The drawing under review shows one solid part. Ordinate dimensions are in mm from its lowest x, y, z. A direction names the side the tool comes from. Coordinates: 2 decimals unless noted, no trailing zeros. Order: outer loops, then holes, each group sorted by start corner. A loop starts at its lowest first (then second) coordinate and runs counter-clockwise, first axis right, second up. Notation, with made-up numbers: (47, 10) - (52, 10) arc R20 cw to (52, 25) - close; hole circle Ø6 at (-9.5, -27). An arc over 180 degrees is marked (long way). Answer in a Markdown table with one row per item.
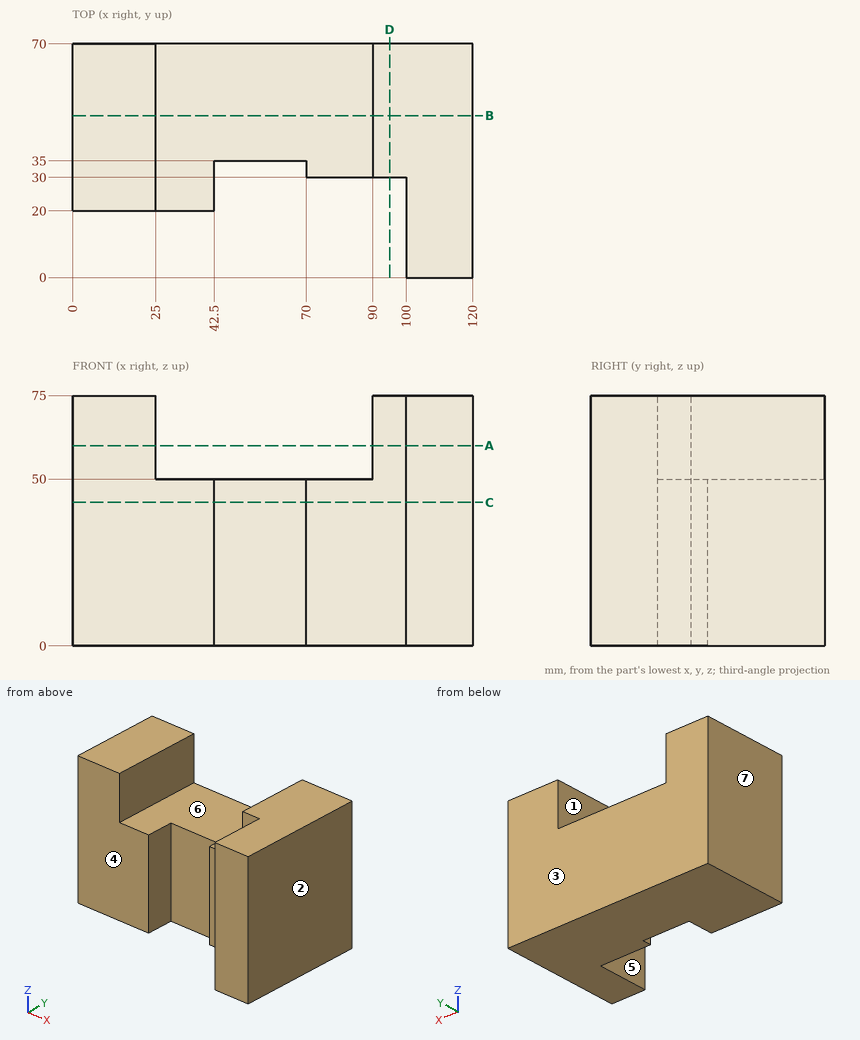
Item 1: We need section B-B, the plane y = 48.5. Write out the cut boundary in (x, z), then the cut area to 4 significant figures.
Check values:
| item | result |
|---|---|
| outline | (0, 0) - (120, 0) - (120, 75) - (90, 75) - (90, 50) - (25, 50) - (25, 75) - (0, 75) - close |
| area | 7,375 mm^2 |
Item 2: Mouldability with a two-part tool opening along X and no side actions: class the marked faces 1, 2 and 3 as +X half, -X half, draft (parallel to the pull), parting line (faces both ways), or undercut.
Check values:
| item | result |
|---|---|
| face 1 | undercut |
| face 2 | +X half |
| face 3 | draft |
Item 3: Tool access review of the marked faces 4, 5, 6 and 7: name each direction out of +Z, -Z, +X, -X, +Y, -Y from which nothing blocks a thin tool from reaching the whole face with its end or side.
Check values:
| item | result |
|---|---|
| face 4 | +Z, -Z, -X, -Y |
| face 5 | +Z, -Z, -Y |
| face 6 | +Z, +Y, -Y |
| face 7 | +Z, -Z, -X, +Y, -Y |
Item 4: We need section C-C, the plane z = 43. Write out the cut boundary in (x, y), then the cut area to 3 significant figures.
Check values:
| item | result |
|---|---|
| outline | (0, 20) - (42.5, 20) - (42.5, 35) - (70, 35) - (70, 30) - (100, 30) - (100, 0) - (120, 0) - (120, 70) - (0, 70) - close |
| area | 5,690 mm^2 |
Item 5: We need section A-A, the plane z = 60. Write out the cut boundary in (x, y).
Check values:
| item | result |
|---|---|
| outline | (0, 20) - (25, 20) - (25, 70) - (0, 70) - close; (90, 30) - (100, 30) - (100, 0) - (120, 0) - (120, 70) - (90, 70) - close |
Item 6: To check wall thickness, follow line 1 (X direction, y = 61.5, z = 71); line 2 (X direction, y = 21, z = 45.5); line 3 (Y direction, x = 19.5, z = 68.5). State the ranges of each line that lie inside material, in increasing order. Write a range as from..to.
Check values:
| item | result |
|---|---|
| line 1 | 0..25, 90..120 |
| line 2 | 0..42.5, 100..120 |
| line 3 | 20..70 |
Item 7: Clearance check with flat-ended pins moving along their axes: pin 1 Ø7.5 at (y, z) = (43.5, 58) entering from -X; pin 2 Ø4 at (x, y) = (68, 61.5) entering from +Z; pin 3 Ø8 at (x, z) = (39.5, 40) entering from -Y; pin 4 Ø1 at (y, z) = (13.5, 17.5) entering from -X. State where each tip first meets the part, or that it passes through.
Check values:
| item | result |
|---|---|
| pin 1 | x = 0 |
| pin 2 | z = 50 |
| pin 3 | y = 20 |
| pin 4 | x = 100 |
Item 8: We need section D-D, the plane x = 95. Write out the cut boundary in (y, z).
Check values:
| item | result |
|---|---|
| outline | (30, 0) - (70, 0) - (70, 75) - (30, 75) - close |
